The model under review builds one solid part; all positions refer to its coordinate system, in mm. Face numbers are marked on the shaded views. A direction names the side the tool comes from. Give positions to 0.01 mm unless a question says otherwise; leave off trailing zeros. Order: outer loops, then holes, each group sorted by start corner. A loop starts at its lowest first (then second) coordinate and runs counter-clockwise, first axis right, second up.
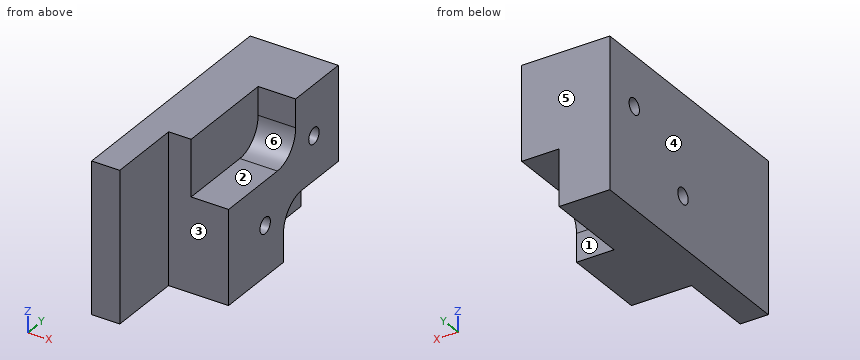
```python
from build123d import *

# Parameters (mm, degrees)
BOSS_EXTRUDE1_DEPTH       = 25.4
TAP_DRILL_FOR_6_32_TAP1_D = 2.7051
SKETCH5_R                 = 4.7625
CUT_EXTRUDE1_DEPTH        = 6.35


with BuildPart() as part:
    # Sketch1 → Boss-Extrude1 (new body)
    with BuildSketch(Plane.XY):
        Polygon((-30.169054899, -23.479397625), (-25.406554899, -23.479397625), (-25.406554899, -10.779397625), (-15.246554899, -10.779397625), (-15.246554899, -7.604397625), (-15.246554899, 17.795602375), (-30.169054899, 17.795602375), (-30.169054899, -7.604397625), align=None)
    extrude(amount=BOSS_EXTRUDE1_DEPTH)

    # Tap Drill for #6-32 Tap1 (through all)
    with Locations(Plane(origin=(-15.246554899, 11.445602375, 16.933333333), x_dir=(0, 1, 0), z_dir=(1, 0, 0))):
        with Locations((0, 0), (-12.7, -8.466666666)):
            Hole(TAP_DRILL_FOR_6_32_TAP1_D / 2)

    # Sketch5 → Cut-Extrude1 (cut)
    with BuildSketch(Plane(origin=(-15.246554899, 0, 0), x_dir=(0, 0, -1), z_dir=(1, 0, 0))):
        with Locations((-20.6375, 1.920602375)):
            Circle(SKETCH5_R)
        with BuildLine():
            ThreePointArc((-25.4, 1.920602382), (-24.005096043, 5.288198423), (-20.6375, 6.683102375))
            Line((-20.6375, 6.683102375), (-25.4, 6.683102375))
            Line((-25.4, 6.683102375), (-25.4, 1.920602382))
        make_face()
        with BuildLine():
            Line((-15.875, -10.779397625), (-15.875, 1.920602375))
            ThreePointArc((-15.875, 1.920602375), (-20.637500004, -2.841897625), (-25.4, 1.920602382))
            Line((-25.4, 1.920602382), (-25.4, -10.779397625))
            Line((-25.4, -10.779397625), (-15.875, -10.779397625))
        make_face()
        with BuildLine():
            Line((0, 17.795602375), (-9.525, 17.795602375))
            Line((-9.525, 17.795602375), (-9.525, 8.270602375))
            ThreePointArc((-9.525, 8.270602375), (-4.7625, 13.033102375), (0, 8.270602375))
            Line((0, 8.270602375), (0, 17.795602375))
        make_face()
        with Locations((-4.7625, 8.270602375)):
            Circle(SKETCH5_R)
        with BuildLine():
            Line((-4.7625, 3.508102375), (0, 3.508102375))
            Line((0, 3.508102375), (0, 8.270602375))
            ThreePointArc((0, 8.270602375), (-1.394903955, 4.90300633), (-4.7625, 3.508102375))
        make_face()
    extrude(amount=-CUT_EXTRUDE1_DEPTH, mode=Mode.SUBTRACT)


solid = part.part
```
Item 1: For line 1 (Z direction, x = -16, y = -7) (3 decimals); line 2 (X direction, y = -12, z = 7.75); line 3 (Y direction, x = -17.25, z = 3.5), list the stretches that pass through material, from the lowest coordinate up.
Values found:
line 1: z = 0 to 15.875
line 2: x = -30.17 to -25.41
line 3: y = -10.78 to 3.51
Item 2: Take a section at C-C (x = -17.5). Give the boundary of the cut face in (y, z) (1 decimal), and give its area (3 significant figures).
Values found:
outline: (-10.8, 0) - (3.5, 0) - (3.5, 4.8) arc R4.8 cw to (8.3, 9.5) - (17.8, 9.5) - (17.8, 25.4) - (6.7, 25.4) - (6.7, 20.6) arc R4.8 cw to (1.9, 15.9) - (-10.8, 15.9) - close; hole circle Ø2.7 at (-1.3, 8.5); hole circle Ø2.7 at (11.4, 16.9)
area: 422 mm2
Item 3: Draft analysis for pull direction Y (two halves, no side actions). For the marked faces 4, 5 and 6, state which applies: released by +Y, released by -Y, zero draft, split by the parting line, or undercut.
Values found:
face 4: zero draft
face 5: released by +Y
face 6: released by -Y
Item 4: For the marked faces 1, 2 and 3, list the 3-axis set-ups (+Z, -Z, +X, -X, +Y, -Y) from which the entire face can be reached by the end or side of a thin tool; tool diameter is ignored.
Values found:
face 1: -Z, +X, +Y
face 2: +Z, +X, -Y
face 3: +Z, -Z, +X, -Y
Item 5: Take a section at B-B (z = 3). Give the boundary of the cut face in (x, y).
Values found:
outline: (-30.17, -23.48) - (-25.41, -23.48) - (-25.41, -10.78) - (-15.25, -10.78) - (-15.25, 3.51) - (-21.6, 3.51) - (-21.6, 17.8) - (-30.17, 17.8) - close
Item 6: Take a section at A-A (y = 11.5). Give the boundary of the cut face in (x, z) (3 decimals), and give its area (3 significant figures).
Values found:
outline: (-30.169, 0) - (-21.597, 0) - (-21.597, 9.525) - (-15.247, 9.525) - (-15.247, 15.582) - (-30.169, 15.582) - close; (-30.169, 18.285) - (-15.247, 18.285) - (-15.247, 25.4) - (-30.169, 25.4) - close
area: 278 mm2
Item 7: Take a section at D-D (y = -15). Give the boundary of the cut face in (x, z).
Values found:
outline: (-30.17, 0) - (-25.41, 0) - (-25.41, 25.4) - (-30.17, 25.4) - close
Item 8: Clearance check with flat-ended pins moving along their axes: pin 1 Ø6 at (x, z) = (-22.5, 22) entering from -Y; pin 2 Ø3 at (x, y) = (-17, 15) entering from -Z (3 decimals); pin 3 Ø5 at (x, z) = (-22.5, 13.5) entering from -Y; pin 4 Ø1.5 at (x, y) = (-18.5, -4.5) entering from +Z (3 decimals). State where each tip first meets the part, or that it passes through.
Values found:
pin 1: stops at y = -23.48
pin 2: stops at z = 9.525
pin 3: stops at y = -10.78
pin 4: stops at z = 15.875
